Geometry: final body of the model. Coordinates: model frame, mm. A direction names the side the tool comes from. Give positions to 0.01 mm unless a question says otherwise; leave off trailing zeros. Write each loop counter-clockwise with the first axis right and the second up, starting at its lowest first coordinate (ties: lowest second). Pieces come first, ordered by that corner, then holes. Notation, with made-up numbers: M -32,-32.75 L -4,-32.75 A19 cw -4,-26.75 Z; hole C -34,3.5 d6. An arc over 180 degrees is marked long. Answer as a JSON object with one key per item and string values.
from build123d import *

# Parameters (mm, degrees)
F1_DEPTH = 510
F3_DEPTH = 27
F5_D     = 6
F7_D     = 12
F7_DEPTH = 4
F7_TIP   = 3.6051637142


with BuildPart() as f1:
    # F0 (on Top) → F1 (new body)
    with BuildSketch(Plane.XY):
        Polygon((-25, 0), (0, 0), (0, 21), (-5, 25.5), (-5, 27), (-20, 27), (-20, 25.5), (-25, 21), align=None)
    extrude(amount=F1_DEPTH)

    # F2 (on face) → F3 (cut)
    with BuildSketch(Plane.XZ):
        with BuildLine():
            ThreePointArc((-25, 506), (-19.0622023742, 508.9756324194), (-12.5, 510))
            Line((-12.5, 510), (-25, 510))
            Line((-25, 510), (-25, 506))
        make_face()
        with BuildLine():
            Line((0, 510), (-12.5, 510))
            ThreePointArc((-12.5, 510), (-5.9377976258, 508.9756324194), (0, 506))
            Line((0, 506), (0, 510))
        make_face()
    extrude(amount=-F3_DEPTH, mode=Mode.SUBTRACT)

    # F5 (through all)
    with Locations(Plane.XZ):
        with Locations((-12.5, 492), (-12.5, 12), (-12.5, 75.6)):
            Hole(F5_D / 2)

    # F7
    with Locations(Plane.XZ):
        with Locations((-12.5, 75.6)):
            Hole(F7_D / 2, depth=F7_DEPTH)
            with Locations((0, 0, -(F7_DEPTH + F7_TIP / 2))):  # 118° drill point
                Cone(0, F7_D / 2, F7_TIP, mode=Mode.SUBTRACT)


solid = f1.part
1) Cut plane A-A on z = 160.5. Return loops of the section in (x, y), and give its area (4 significant figures).
Geometry check:
{"outline": "M -25,0 L 0,0 L 0,21 L -5,25.5 L -5,27 L -20,27 L -20,25.5 L -25,21 Z", "area": "637.5 mm2"}
2) Set-up query: faces 4 (the cylindrical face through (-11.72, 2.03, 81.55)), 5 (the flat face through (-13, 0, 251)). Return all of +Z, -Z, +X, -X, +Y, -Y with unobstructed straight access to the full face (end or side cutting, diameter ignored); none if empty.
Geometry check:
{"face 4": "-Y", "face 5": "+Z, -Z, +X, -X, -Y"}
3) Contact query for flat-ended pins moving along their axis: P1, Ø8, axis at x = -16, y = 3.5, coming from the -Z side; P2, Ø0.8, axis at y = 26, z = 227.5, coming from the -X side; P3, Ø8, axis at x = -12.5, z = 75.6, coming from the -Y side; P4, Ø8, axis at x = -8, y = 22.5, coming from the +Z side. Output: stop coordinate, or through.
Geometry check:
{"P1": "stops at z = 0", "P2": "stops at x = -20", "P3": "stops at y = 5.2", "P4": "stops at z = 509.99"}
4) Line query: line 1 (Z direction, x = -12.5, y = 13.5); line 2 (Z direction, x = -10.5, y = 18.25); line 3 (X direction, y = 9, z = 492). Output: solid intervals per line, ascending. Write a range as from..to.
Geometry check:
{"line 1": "z = 0..9, 15..72.6, 78.6..489, 495..510", "line 2": "z = 0..9.76, 14.24..73.36, 77.84..489.76, 494.24..509.91", "line 3": "x = -25..-15.5, -9.5..0"}
5) Pull-direction query (Z, two-part tool) for faces 1 (the flat face through (-12, 27, 251)), 2 (the conical face through (-11.03, 5.69, 72.77)), 3 (the flat face through (-13, 14, 0)); classes: pulls with the +Z half, pulls with the -Z half, needs draft (parallel to the pull), parting line crosses it, or undercut.
Geometry check:
{"face 1": "needs draft", "face 2": "undercut", "face 3": "pulls with the -Z half"}
